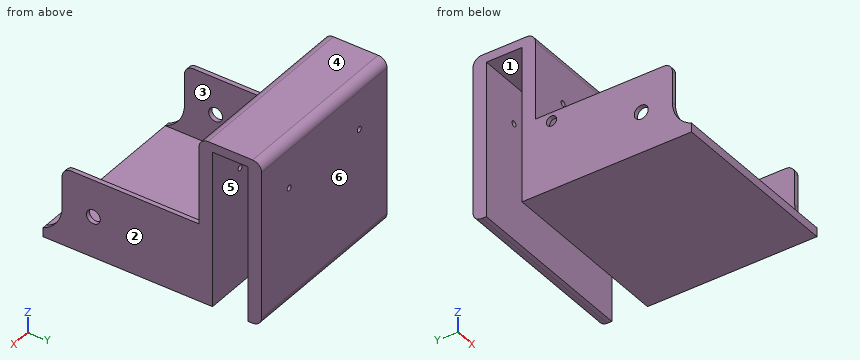
```python
from build123d import *

# Parameters (mm, degrees)
F0_W        = 7.62
F0_H        = 88.9
F0_H_2      = 83.82
F0_W_2      = 88.9
F0_H_3      = 5.08
F1_DEPTH    = 101.6
F3_START    = 17.018
F3_DEPTH    = 78.74
F4_T1_DEPTH = 2.54
F4_T3_DEPTH = 2.54
F5_R        = 5.08
F6_R        = 5.08
F7_R        = 5.08
F8_R        = 3.9711233586
F9_DEPTH    = 154.686
F10_R       = 2.8797148657
F11_DEPTH   = 33.782
F12_R       = 1.5875
F13_DEPTH   = 85.344


# Not quite as in the source:
# - a fillet or chamfer that OpenCascade refuses, or shapes differently, is made with other operations: its cross-section is extruded or revolved along the edge and cut away or added


with BuildPart() as f1:
    # F0 (on Right) → F1 (new body)
    with BuildSketch(Plane.YZ):
        with Locations((13.97, 0)):
            Rectangle(F0_W, F0_H)
        Polygon((-10.16, 44.45), (10.16, 44.45), (17.78, 44.45), (17.78, 49.53), (-17.78, 49.53), (-17.78, 44.45), align=None)
        with Locations((-13.97, 2.54)):
            Rectangle(F0_W, F0_H_2)
        with Locations((-62.23, -41.91)):
            Rectangle(F0_W_2, F0_H_3)
        with Locations((-13.97, -41.91)):
            Rectangle(F0_W, F0_H_3)
    extrude(amount=F1_DEPTH)

    # F2 (on Front) → F3 (join)
    with BuildSketch(Plane.XZ.offset(F3_START)):
        Polygon((0, 0), (0, -39.37), (0, -44.45), (2.54, -44.45), (2.54, 0), align=None)
        Polygon((101.6, 0), (99.06, 0), (99.06, -44.45), (101.6, -44.45), (101.6, -39.37), align=None)
    extrude(amount=F3_DEPTH)

    # F4: fillet of radius 17.78 on 2 edges, made by hand

    # F4_s2 → F4_t1 (join)
    with BuildSketch(Plane.YZ.offset(99.06)):
        with BuildLine():
            ThreePointArc((-106.68, -39.37), (-98.7382763539, -32.8196066778), (-95.758, -22.9658469893))
            Line((-95.758, -22.9658469893), (-95.758, -39.37))
            Line((-95.758, -39.37), (-106.68, -39.37))
        make_face()
    extrude(amount=F4_T1_DEPTH)

    # F4_s4 → F4_t3 (join)
    with BuildSketch(Plane.YZ):
        with BuildLine():
            ThreePointArc((-106.68, -39.37), (-98.7382763539, -32.8196066778), (-95.758, -22.9658469893))
            Line((-95.758, -22.9658469893), (-95.758, -39.37))
            Line((-95.758, -39.37), (-106.68, -39.37))
        make_face()
    extrude(amount=F4_T3_DEPTH)

    # F5
    f5_edges = [f1.edges().sort_by_distance(p)[0] for p in [
        (1.27, -95.758, 0),
        (100.33, -95.758, 0),
    ]]
    fillet(f5_edges, radius=F5_R)

    # F6
    f6_edges = [f1.edges().sort_by_distance(p)[0] for p in [
        (50.8, -17.78, 49.53),
        (50.8, 17.78, 49.53),
    ]]
    fillet(f6_edges, radius=F6_R)

    # F7
    f7_edges = [f1.edges().sort_by_distance(p)[0] for p in [
        (50.8, 17.78, -44.45),
    ]]
    fillet(f7_edges, radius=F7_R)

    # F8 (on Right) → F9 (cut)
    with BuildSketch(Plane.YZ):
        with Locations((-78.0128240585, -21.108629182)):
            Circle(F8_R)
    extrude(amount=F9_DEPTH, mode=Mode.SUBTRACT)

    # F10 (on Right) → F11 (cut)
    with BuildSketch(Plane.YZ):
        with Locations((-26.9465316087, -4.8854034394)):
            Circle(F10_R)
    extrude(amount=F11_DEPTH, mode=Mode.SUBTRACT)

    # F12 (on face) → F13 (cut)
    with BuildSketch(Plane.XZ.offset(17.78)):
        with Locations((22.3786290735, 22.225)):
            Circle(F12_R)
        with Locations((79.2213709265, 22.225)):
            Circle(F12_R)
    extrude(amount=-F13_DEPTH, mode=Mode.SUBTRACT)


solid = f1.part
```
Geometry: final body of the model. Coordinates: model frame, mm. Face numbers are marked on the shaded views. A direction names the side the tool comes from. Round coordinates to 2 decimals unless told otherwise and drop trailing zeros. Write each loop counter-clockwise with the first axis right and the second up, starting at its lowest first coordinate (ties: lowest second). Pieces come first, ordered by that corner, then holes. Notation, with made-up numbers: M 29.5,12.25 L 52.5,12.25 A15 cw 52.5,37.25 Z; hole C 2,37 d7. An arc over 180 degrees is marked long. Answer in a Markdown table with one row per item. Add a question column.
(1) Reachability of the marked faces 1, 2 and 3 from +Z, -Z, +X, -X, +Y, -Y: full face, straight path, thin tool, end or side. Return the list, or none.
(2) Cut plane A-A, the plane z = -9.5. Return the cut outline in (x, y), then the cut area to 3 significant figures.
(3) Draft query along Y for the marked faces 4, 5 and 6. Return one class per face: pulls with the +Y half, pulls with the -Y half, needs draft (parallel to the pull), parting line crosses it, or undercut.
(4) Contact query for flat-ended pins moving along their axis: pin 1 (3 mm diameter, centred on x = 88.5, y = -20.5, fed in from +Z); pin 2 (1.3 mm diameter, centred on x = 1.5, z = -10, fed in from -Y); pin 3 (1.3 mm diameter, centred on x = 100.5, y = -61.5, fed in from +Z). Output: stop coordinate, or through.
(5) Cut plane C-C, the plane y = -77.5. Return the cut outline in (x, z), then the cut area to 3 significant figures.
(6) Ray query, L1, parallel to Y at x = 13.5, z = 23.5; L2, parallel to X at y = -61.5, z = -19.5; L3, parallel to Z at x = 40.5, y = -76.5. Return the intervals inside material, ascending.
(7) Cut plane B-B, the plane y = -26. Return the cut outline in (x, z), then the cut area to 3 significant figures.
(8) Cut plane D-D, the plane x = 49. Return the cut outline in (y, z), then the cut area to 3 significant figures.
Established:
| question | item | result |
|---|---|---|
| 1 | face 1 | -Z, +X, -X |
| 1 | face 2 | +Z, -Z, +X, +Y, -Y |
| 1 | face 3 | +Z, -Y |
| 2 | outline | M 0,-95.76 L 2.54,-95.76 L 2.54,-17.78 L 99.06,-17.78 L 99.06,-95.76 L 101.6,-95.76 L 101.6,-10.16 L 0,-10.16 Z; M 0,10.16 L 101.6,10.16 L 101.6,17.78 L 0,17.78 Z |
| 2 | area | 1,940 mm² |
| 3 | face 4 | needs draft |
| 3 | face 5 | undercut |
| 3 | face 6 | pulls with the +Y half |
| 4 | pin 1 | z = -39.37 |
| 4 | pin 2 | y = -95.76 |
| 4 | pin 3 | z = 0 |
| 5 | outline | M 0,-44.45 L 101.6,-44.45 L 101.6,-25.05 L 99.06,-25.05 L 99.06,-39.37 L 2.54,-39.37 L 2.54,-25.05 L 0,-25.05 Z; M 0,-17.17 L 2.54,-17.17 L 2.54,0 L 0,0 Z; M 99.06,-17.17 L 101.6,-17.17 L 101.6,0 L 99.06,0 Z |
| 5 | area | 676 mm² |
| 6 | L1 | -17.78 to -10.16, 10.16 to 17.78 |
| 6 | L2 | 0 to 2.54, 99.06 to 101.6 |
| 6 | L3 | -44.45 to -39.37 |
| 7 | outline | M 0,-44.45 L 101.6,-44.45 L 101.6,0 L 99.06,0 L 99.06,-39.37 L 2.54,-39.37 L 2.54,-7.61 L 0,-7.61 Z; M 0,-2.17 L 2.54,-2.17 L 2.54,0 L 0,0 Z |
| 7 | area | 702 mm² |
| 8 | outline | M -106.68,-44.45 L -10.16,-44.45 L -10.16,44.45 L 10.16,44.45 L 10.16,-44.45 L 12.7,-44.45 A5.08 ccw 17.78,-39.37 L 17.78,44.45 A5.08 ccw 12.7,49.53 L -12.7,49.53 A5.08 ccw -17.78,44.45 L -17.78,-39.37 L -106.68,-39.37 Z |
| 8 | area | 1,970 mm² |
